Can you work these out from the model? Positions are in its coordinate system, mm. A direction names the side the tool comes from. Coordinates: 2 decimals unless noted, no trailing zeros. Order: outer loops, then holes, each group sorted by start corner. A loop starts at its lowest first (then second) coordinate and runs counter-clockwise, first axis right, second up. Notation, with made-up numbers: (25, -12) -> (68, -12) arc R18 cw to (68, -3) -> close; hole circle Ø11 at (-10, -18). An arc over 180 degrees is marked (long way). Use a Markdown table: item, result. Add a question column.
1. Suppose I cut it at B-B, the plane z = 0. List the corners of the cut face in (x, y) for me, then the cut area to 3 significant figures.
2. Suppose I cut it at C-C, the plane z = -32. List the corners of the cut face in (x, y) for me.
3. If I drill on line 1 along Y through (x, z) = (4.7, 0); line 2 along Y through (x, z) = (5.7, 1.5); line 3 along Z through (x, y) = (2.2, 3.5), over which ranges is the centre line in solid material (lowest first)? Write a range as from..to.
4. For pin 1 Ø1.8 at (x, z) = (1.5, 2.5) entering from +Y; pin 2 Ø1.8 at (x, z) = (2.5, -4.5) entering from -Y; pin 3 Ø3 at (x, y) = (3, 2.5) entering from +Z; pin 4 Ø8 at (y, z) = (0, 32) entering from +X, each with a flat end and sliding along its axis, tell me the tip position at first contact or that it passes through.
5. Suppose I cut it at A-A, the plane y = 0. List the corners of the cut face in (x, z) for me, then the cut area to 3 significant figures.
6. We'd pull the mould along Y, two halves only. Please class faces 3 (the cylindrical face through (2.958, -28.751, 37.496)), 4 (the flat face through (0, -20, 1)), 5 (the flat face through (3, 15.15, 0)): pulls with the +Y half, pulls with the -Y half, needs draft (parallel to the pull), parting line crosses it, or undercut.
7. For faces 1 (the flat face through (3, 1, -13)), 2 (the flat face through (6, -20, 1)), which set-ups out of +Z, -Z, +X, -X, +Y, -Y let a thin tool reach every point of the face, with its end or its side?
```python
from build123d import *

# Parameters (mm, degrees)
SKETCH1_R                                           = 47.25
BOSS_EXTRUDE1_DEPTH                                 = 6
CUT_EXTRUDE1_DEPTH                                  = 20
CBORE_FOR_M5_HEX_SOCKET_HEAD_CAP_SCREW2_D           = 5.3
CBORE_FOR_M5_HEX_SOCKET_HEAD_CAP_SCREW2_DEPTH       = 20
CBORE_FOR_M5_HEX_SOCKET_HEAD_CAP_SCREW2_CBORE_D     = 10
CBORE_FOR_M5_HEX_SOCKET_HEAD_CAP_SCREW2_CBORE_DEPTH = 15.4
CBORE_FOR_M5_HEX_SOCKET_HEAD_CAP_SCREW2_TIP         = 1.59228064


with BuildPart() as part:
    # Sketch1 → Boss-Extrude1 (new body)
    with BuildSketch(Plane(origin=(0, 0, 0), x_dir=(0, 0, -1), z_dir=(1, 0, 0))):
        Circle(SKETCH1_R)
    extrude(amount=BOSS_EXTRUDE1_DEPTH)

    # Sketch2 → Cut-Extrude1 (cut)
    with BuildSketch(Plane(origin=(6, 0, 0), x_dir=(0, 0, -1), z_dir=(1, 0, 0))):
        with BuildLine():
            Line((-12, -12.85), (12, -12.85))
            ThreePointArc((12, -12.85), (12.707106781, -12.557106781), (13, -11.85))
            Line((13, -11.85), (13, -10.85))
            ThreePointArc((13, -10.85), (12.707106781, -11.557106781), (12, -11.85))
            Line((12, -11.85), (-12, -11.85))
            ThreePointArc((-12, -11.85), (-12.707106781, -11.557106781), (-13, -10.85))
            Line((-13, -10.85), (-13, -11.85))
            ThreePointArc((-13, -11.85), (-12.707106781, -12.557106781), (-12, -12.85))
        make_face()
        with BuildLine():
            ThreePointArc((12, -11.85), (12.707106781, -11.557106781), (13, -10.85))
            Line((13, -10.85), (13, -3.85))
            Line((13, -3.85), (13, 14.15))
            ThreePointArc((13, 14.15), (12.707106781, 14.857106781), (12, 15.15))
            Line((12, 15.15), (-12, 15.15))
            ThreePointArc((-12, 15.15), (-12.707106781, 14.857106781), (-13, 14.15))
            Line((-13, 14.15), (-13, -3.85))
            Line((-13, -3.85), (-13, -10.85))
            ThreePointArc((-13, -10.85), (-12.707106781, -11.557106781), (-12, -11.85))
            Line((-12, -11.85), (12, -11.85))
        make_face()
    extrude(amount=-CUT_EXTRUDE1_DEPTH, mode=Mode.SUBTRACT)

    # CBORE for M5 Hex Socket Head Cap Screw2
    with Locations(Plane.ZY):
        with Locations((-32, 0), (0, 32), (32, 0), (0, -32)):
            CounterBoreHole(CBORE_FOR_M5_HEX_SOCKET_HEAD_CAP_SCREW2_D / 2, CBORE_FOR_M5_HEX_SOCKET_HEAD_CAP_SCREW2_CBORE_D / 2, CBORE_FOR_M5_HEX_SOCKET_HEAD_CAP_SCREW2_CBORE_DEPTH, depth=CBORE_FOR_M5_HEX_SOCKET_HEAD_CAP_SCREW2_DEPTH)
            with Locations((0, 0, -(CBORE_FOR_M5_HEX_SOCKET_HEAD_CAP_SCREW2_DEPTH + CBORE_FOR_M5_HEX_SOCKET_HEAD_CAP_SCREW2_TIP / 2))):  # 118° drill point
                Cone(0, CBORE_FOR_M5_HEX_SOCKET_HEAD_CAP_SCREW2_D / 2, CBORE_FOR_M5_HEX_SOCKET_HEAD_CAP_SCREW2_TIP, mode=Mode.SUBTRACT)


solid = part.part
```
Worked out:
| question | item | result |
|---|---|---|
| 1 | outline | (0, -47.25) -> (6, -47.25) -> (6, -37) -> (0, -37) -> close; (0, -27) -> (6, -27) -> (6, -12.85) -> (0, -12.85) -> close; (0, 15.15) -> (6, 15.15) -> (6, 27) -> (0, 27) -> close; (0, 37) -> (6, 37) -> (6, 47.25) -> (0, 47.25) -> close |
| 1 | area | 279 mm² |
| 2 | outline | (0, -34.76) -> (6, -34.76) -> (6, -5) -> (0, -5) -> close; (0, 5) -> (6, 5) -> (6, 34.76) -> (0, 34.76) -> close |
| 3 | line 1 | y = -47.25..-37, -27..-12.85, 15.15..27, 37..47.25 |
| 3 | line 2 | y = -47.23..-36.77, -27.23..-12.85, 15.15..27.23, 36.77..47.23 |
| 3 | line 3 | z = -47.12..-35.57, -28.43..-13, 13..28.43, 35.57..47.12 |
| 4 | pin 1 | stops at y = 47.22 |
| 4 | pin 2 | stops at y = -47.11 |
| 4 | pin 3 | stops at z = 47.24 |
| 4 | pin 4 | passes through |
| 5 | outline | (0, -47.25) -> (6, -47.25) -> (6, -37) -> (0, -37) -> close; (0, -27) -> (6, -27) -> (6, -13) -> (0, -13) -> close; (0, 13) -> (6, 13) -> (6, 27) -> (0, 27) -> close; (0, 37) -> (6, 37) -> (6, 47.25) -> (0, 47.25) -> close |
| 5 | area | 291 mm² |
| 6 | face 3 | parting line crosses it |
| 6 | face 4 | needs draft |
| 6 | face 5 | undercut |
| 7 | face 1 | +X, -X |
| 7 | face 2 | +Z, -Z, +X, +Y, -Y |
